```python
from build123d import *

# Parameters (mm, degrees)
SKETCH1_R           = 11
BOSS_EXTRUDE1_DEPTH = 3
SKETCH2_R           = 6
BOSS_EXTRUDE2_DEPTH = 20
CUT_EXTRUDE1_DEPTH  = 15


with BuildPart() as part:
    # Sketch1 → Boss-Extrude1 (new body)
    with BuildSketch(Plane.XY):
        Circle(SKETCH1_R)
    extrude(amount=BOSS_EXTRUDE1_DEPTH)

    # Sketch2 → Boss-Extrude2 (add)
    with BuildSketch(Plane.XY.offset(3)):
        Circle(SKETCH2_R)
    extrude(amount=BOSS_EXTRUDE2_DEPTH)

    # Sketch3 → Cut-Extrude1 (cut)
    with BuildSketch(Plane.XY.offset(23)):
        with BuildLine():
            Line((-3.5, 4.873397172), (-3.5, -4.873397172))
            ThreePointArc((-3.5, -4.873397172), (-6, 0), (-3.5, 4.873397172))
        make_face()
    extrude(amount=-CUT_EXTRUDE1_DEPTH, mode=Mode.SUBTRACT)


solid = part.part
```
The model under review builds one solid part; all positions refer to its coordinate system, in mm. A direction names the side the tool comes from. Give positions to 0.01 mm unless a question says otherwise; leave off trailing zeros. Write each loop counter-clockwise with the first axis right and the second up, starting at its lowest first coordinate (ties: lowest second). Pieces come first, ordered by that corner, then holes. Notation, with made-up numbers: (37, -34) -> (92, -34) arc R7 cw to (92, -24) -> close; hole circle Ø9 at (76.5, -14.5). An arc over 180 degrees is marked (long way). Answer in a Markdown table with one row per item.
1) Tool access review of faces 1 (the flat face through (-3.5, 0, 16)), 2 (the flat face through (0, 0, 0)), 3 (the cylindrical face through (5.723, 1.802, 12.86)): name each direction out of +Z, -Z, +X, -X, +Y, -Y from which nothing blocks a thin tool from reaching the whole face with its end or side.
Worked answers:
| item | result |
|---|---|
| face 1 | +Z, -X, +Y, -Y |
| face 2 | -Z, +X, -X, +Y, -Y |
| face 3 | +Z |
2) Clearance check with flat-ended pins moving along their axes: P1, Ø1, axis at x = -4, y = 7, coming from the +Z side; P2, Ø12, axis at x = 7.5, z = 18.5, coming from the +Y side; P3, Ø8, axis at y = 5, z = 11, coming from the -X side. State where each tip first meets the part, or that it passes through.
Worked answers:
| item | result |
|---|---|
| P1 | z = 3 |
| P2 | y = 5.81 |
| P3 | x = -5.52 |
3) Add section C-C on z = 13. State the section outline as (x, y) points.
Worked answers:
| item | result |
|---|---|
| outline | (-3.5, -4.87) arc R6 ccw (long way) to (-3.5, 4.87) -> close |
4) Add section A-A on y = 0. State the section outline as (x, z) points.
Worked answers:
| item | result |
|---|---|
| outline | (-11, 0) -> (11, 0) -> (11, 3) -> (6, 3) -> (6, 23) -> (-3.5, 23) -> (-3.5, 8) -> (-6, 8) -> (-6, 3) -> (-11, 3) -> close |
5) Add section B-B on x = 0. State the section outline as (y, z) points, plus the area to 3 significant figures.
Worked answers:
| item | result |
|---|---|
| outline | (-11, 0) -> (11, 0) -> (11, 3) -> (6, 3) -> (6, 23) -> (-6, 23) -> (-6, 3) -> (-11, 3) -> close |
| area | 306 mm² |
6) Add section D-D on x = 3.5. State the section outline as (y, z) points, plus the area to 3 significant figures.
Worked answers:
| item | result |
|---|---|
| outline | (-10.43, 0) -> (10.43, 0) -> (10.43, 3) -> (4.87, 3) -> (4.87, 23) -> (-4.87, 23) -> (-4.87, 3) -> (-10.43, 3) -> close |
| area | 258 mm² |
7) For L1, parallel to Z at x = -3, y = -6; L2, parallel to X at y = 3.75, z = 17; L3, parallel to X at y = 5.5, z = 2.5, list the stretches that pass through material, from the lowest coordinate up. Write a range as [from, to].
Worked answers:
| item | result |
|---|---|
| L1 | [0, 3] |
| L2 | [-3.5, 4.68] |
| L3 | [-9.53, 9.53] |
